from build123d import *

# Parameters (mm, degrees)
SKETCH2_W          = 15.226765086
SKETCH2_H          = 1.5875
CUT_EXTRUDE1_DEPTH = 85.496179975
FILLET1_R          = 3.175


with BuildPart() as part:
    # Sketch1 → Revolve1 (revolve)
    with BuildSketch(Plane.XY, mode=Mode.PRIVATE) as revolve1_sk:
        Polygon((0, 19.05), (0, 12.7), (80.0862, 12.7), (80.0862, 15.875), (76.9112, 15.875), (76.9112, 14.9098), (74.295, 14.9098), (74.295, 15.875), (3.175, 15.875), (3.175, 19.05), align=None)
    revolve(revolve1_sk.sketch.rotate(Axis((0, 0, 0), (1, 0, 0)), 90), axis=Axis((0, 0, 0), (1, 0, 0)))

    # Sketch2 → Cut-Extrude1 (cut, through all)
    with BuildSketch(Plane.ZY):
        with Locations((0, 18.25625)):
            Rectangle(SKETCH2_W, SKETCH2_H)
        with Locations((0, -18.25625)):
            Rectangle(SKETCH2_W, SKETCH2_H)
    extrude(amount=-CUT_EXTRUDE1_DEPTH, mode=Mode.SUBTRACT)

    # Fillet1
    fillet1_edges = [part.edges().sort_by_distance(p)[0] for p in [
        (1.5875, 17.4625, 7.613382543),
        (1.5875, 17.4625, -7.613382543),
        (1.5875, -17.4625, -7.613382543),
        (1.5875, -17.4625, 7.613382543),
    ]]
    fillet(fillet1_edges, radius=FILLET1_R)


solid = part.part
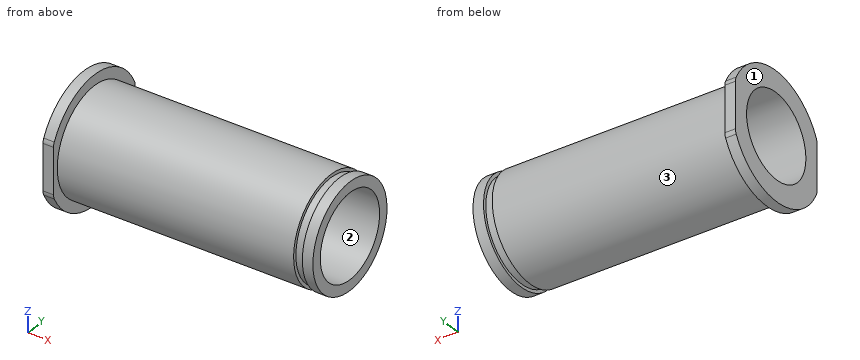
Model file for the job. Use its own axes, mm. Face numbers are marked on the shaded views. Give positions to 0.01 mm unless a question says otherwise; leave off trailing zeros. Loops run counter-clockwise (first coordinate to the right, second up) from the corner with the lowest first, then second, coordinate; pieces in that order, holes last.
1) Saw through at B-B (y = 0). Write the cut outline in (x, z) (3 decimals), plus the area to 3 significant figures.
2) Saw through at C-C (x = 33.5). Write the cut outline in (y, z) (3 decimals), plus the area to 3 significant figures.
3) Saw through at A-A (z = 0). Write the cut outline in (x, y) (1 decimal).
4) Flat gauge pins, fed straight in: pin 1 Ø6 at (x, y) = (21, -8.5) entering from -Z; pin 2 Ø4 at (x, z) = (37, 1) entering from -Y (3 decimals); pin 3 Ø10 at (x, z) = (60.5, 0) entering from +Y (3 decimals). Where does each tip first touch, or does it go through?
5) Wall check: line 1 (X direction, y = -9, z = 12) (3 decimals); line 2 (Z direction, x = 8, y = -0.5); line 3 (Y direction, x = 52, z = 0) (3 decimals). Give the ranges that are in metal, low to high.
6) Pull direction Z, two halves, no side cores. Call the marked faces 1, 2 and 3: +Z half, -Z half, draft (parallel to the pull), parting line (faces both ways), or undercut.
Answer block:
1. outline: (0, -19.05) - (3.175, -19.05) - (3.175, -15.875) - (74.295, -15.875) - (74.295, -14.91) - (76.911, -14.91) - (76.911, -15.875) - (80.086, -15.875) - (80.086, -12.7) - (0, -12.7) - close; (0, 12.7) - (80.086, 12.7) - (80.086, 15.875) - (76.911, 15.875) - (76.911, 14.91) - (74.295, 14.91) - (74.295, 15.875) - (3.175, 15.875) - (3.175, 19.05) - (0, 19.05) - close
1. area: 524 mm2
2. outline: circle Ø31.75 at (0, 0); hole circle Ø25.4 at (0, 0)
2. area: 285 mm2
3. outline: (0, -17.5) - (3.2, -17.5) - (3.2, -15.9) - (74.3, -15.9) - (74.3, -14.9) - (76.9, -14.9) - (76.9, -15.9) - (80.1, -15.9) - (80.1, -12.7) - (0, -12.7) - close; (0, 12.7) - (80.1, 12.7) - (80.1, 15.9) - (76.9, 15.9) - (76.9, 14.9) - (74.3, 14.9) - (74.3, 15.9) - (3.2, 15.9) - (3.2, 17.5) - (0, 17.5) - close
4. pin 1: stops at z = -14.89
4. pin 2: stops at y = -15.875
4. pin 3: stops at y = 15.875
5. line 1: x = 0 to 74.295, 76.911 to 80.086
5. line 2: z = -15.87 to -12.69, 12.69 to 15.87
5. line 3: y = -15.875 to -12.7, 12.7 to 15.875
6. face 1: draft
6. face 2: undercut
6. face 3: parting line
